Part model, mm, in its own coordinate system. A direction names the side the tool comes from. Coordinates: 2 decimals unless noted, no trailing zeros. Loops run counter-clockwise (first coordinate to the right, second up) from the corner with the lowest first, then second, coordinate; pieces in that order, holes last. Notation, with made-up numbers: (23.25, 75.5) -> (60.25, 75.5) arc R31 ccw to (60.25, 107.5) -> close; hole circle Ø4 at (76, 22.5). An arc over 180 degrees is marked (long way). Use one line per item in the form item = value. Start each with the question number.
(1) Pin check, flat tips, straight feed: P1, Ø1, axis at y = -6.5, z = 0.5, coming from the -X side; P2, Ø3, axis at x = 0.5, z = 0, coming from the +Y side; P3, Ø1.5, axis at x = 0, y = -5, coming from the +Z side. Stop position of each tip, or through.
(2) 3-axis set-ups, long thin cutter, end or side, ignore diameter. For faces 1 (the flat face through (-1.413, 1.507, -0.007)), 2 (the flat face through (-1, 0, 1)), 3 (the flat face through (-1, 2, 1)): which of +Z, -Z, +X, -X, +Y, -Y reach the whole face in a straight line?
(3) Drill centre lines: L1, parallel to Y at x = -0.85, z = 0.8; L2, parallel to Z at x = -0.1, y = 0.5; L3, parallel to X at y = -4.75, z = 0. Where is each one in solid material? Low to high. Write a range as [from, to].
(4) Band-saw the part on A-A on y = 0.5. Give the cut face in (x, z), then the cut area to 3 significant figures.
(5) Mould opens along Z. For faces 4 (the flat face through (0, -7.5, 0)), 5 (the cylindrical face through (1, -4, 0)), 6 (the flat face through (-0.904, 1.507, -0.413)) say: +Z half, -Z half, draft (parallel to the pull), parting line (faces both ways), or undercut.
```python
from build123d import *

# Parameters (mm, degrees)
SKETCH1_R           = 2.75
BOSS_EXTRUDE1_DEPTH = 2
FILLET1_SIZE        = 0.2
FILLET1_SIZE_2      = 1
SKETCH2_R           = 1
BOSS_EXTRUDE2_DEPTH = 7.5
CUT_EXTRUDE1_DEPTH  = 1
CUT_EXTRUDE1_DRAFT  = -10


with BuildPart() as part:
    # Sketch1 → Boss-Extrude1 (new body)
    with BuildSketch(Plane(origin=(0, 0, 0), x_dir=(1, 0, 0), z_dir=(0, 1, 0))):
        with Locations(Location((0, 0, 0), (0, 0, 270))):
            Circle(SKETCH1_R)
    extrude(amount=BOSS_EXTRUDE1_DEPTH)

    # Fillet1
    # an asymmetric fillet: 1, 0.2 mm, written as the material it takes off along each edge
    with BuildSketch(Plane(origin=(0, 0, 0), x_dir=(0, 0, 1), z_dir=(-1, 0, 0))) as fillet1_piece_1:
        with BuildLine():
            Bezier((2.75, FILLET1_SIZE), (2.75, 0), (2.75 - FILLET1_SIZE_2, 0), weights=[1, 0.707106781, 1])
            Line((2.75 - FILLET1_SIZE_2, 0), (2.75, 0))
            Line((2.75, 0), (2.75, FILLET1_SIZE))
        make_face()
    revolve(axis=Axis((0, 0, 0), (0, 1, 0)), mode=Mode.SUBTRACT)
    with BuildSketch(Plane(origin=(0, 2, 0), x_dir=(0, 0, 1), z_dir=(-1, 0, 0))) as fillet1_piece_2:
        with BuildLine():
            Bezier((2.75, -FILLET1_SIZE_2), (2.75, 0), (2.75 - FILLET1_SIZE, 0), weights=[1, 0.707106781, 1])
            Line((2.75 - FILLET1_SIZE, 0), (2.75, 0))
            Line((2.75, 0), (2.75, -FILLET1_SIZE_2))
        make_face()
    revolve(axis=Axis((0, 2, 0), (0, 1, 0)), mode=Mode.SUBTRACT)

    # Sketch2 → Boss-Extrude2 (add)
    with BuildSketch(Plane.XZ):
        with Locations(Location((0, 0, 0), (0, 0, 90))):
            Circle(SKETCH2_R)
    extrude(amount=BOSS_EXTRUDE2_DEPTH)


with BuildPart() as cut_extrude1_tool:
    # Sketch5 → Cut-Extrude1 (with draft: the straight prism first)
    with BuildSketch(Plane(origin=(0, 2, 0), x_dir=(1, 0, 0), z_dir=(0, 1, 0))):
        Polygon((0.5, 0.5), (0.5, 1.5), (-0.5, 1.5), (-0.5, 0.5), (-1.5, 0.5), (-1.5, -0.5), (-0.5, -0.5), (-0.5, -1.5), (0.5, -1.5), (0.5, -0.5), (1.5, -0.5), (1.5, 0.5), align=None)
    extrude(amount=-CUT_EXTRUDE1_DEPTH)
    # Cut-Extrude1: the draft: its side faces are tilted about the plane it starts from
    cut_extrude1_sides = [cut_extrude1_tool.faces().sort_by_distance(p)[0] for p in [
        (0.5, 1.5, -1),
        (0, 1.5, -1.5),
        (-0.5, 1.5, -1),
        (-1, 1.5, -0.5),
        (-1.5, 1.5, 0),
        (-1, 1.5, 0.5),
        (-0.5, 1.5, 1),
        (0, 1.5, 1.5),
        (0.5, 1.5, 1),
        (1, 1.5, 0.5),
        (1.5, 1.5, 0),
        (1, 1.5, -0.5),
    ]]
    draft(cut_extrude1_sides, Plane(origin=(0, 2, 0), x_dir=(1, 0, 0), z_dir=(0, 1, 0)), CUT_EXTRUDE1_DRAFT)


with BuildPart() as part_1:
    add(part.part)

    # Cut-Extrude1: cut by cut_extrude1_tool
    add(cut_extrude1_tool.part, mode=Mode.SUBTRACT)


solid = part_1.part
```
A:
q1.P1 = -1
q1.P2 = 2
q1.P3 = 1
q2.face_1 = +Y
q2.face_2 = -Y
q2.face_3 = +Z, -Z, +X, -X, +Y
q3.L1 = [0, 2]
q3.L2 = [-2.75, 2.75]
q3.L3 = [-1, 1]
q4.outline = circle Ø5.5 at (0, 0)
q4.area = 23.8 mm²
q5.face_4 = draft
q5.face_5 = parting line
q5.face_6 = undercut
